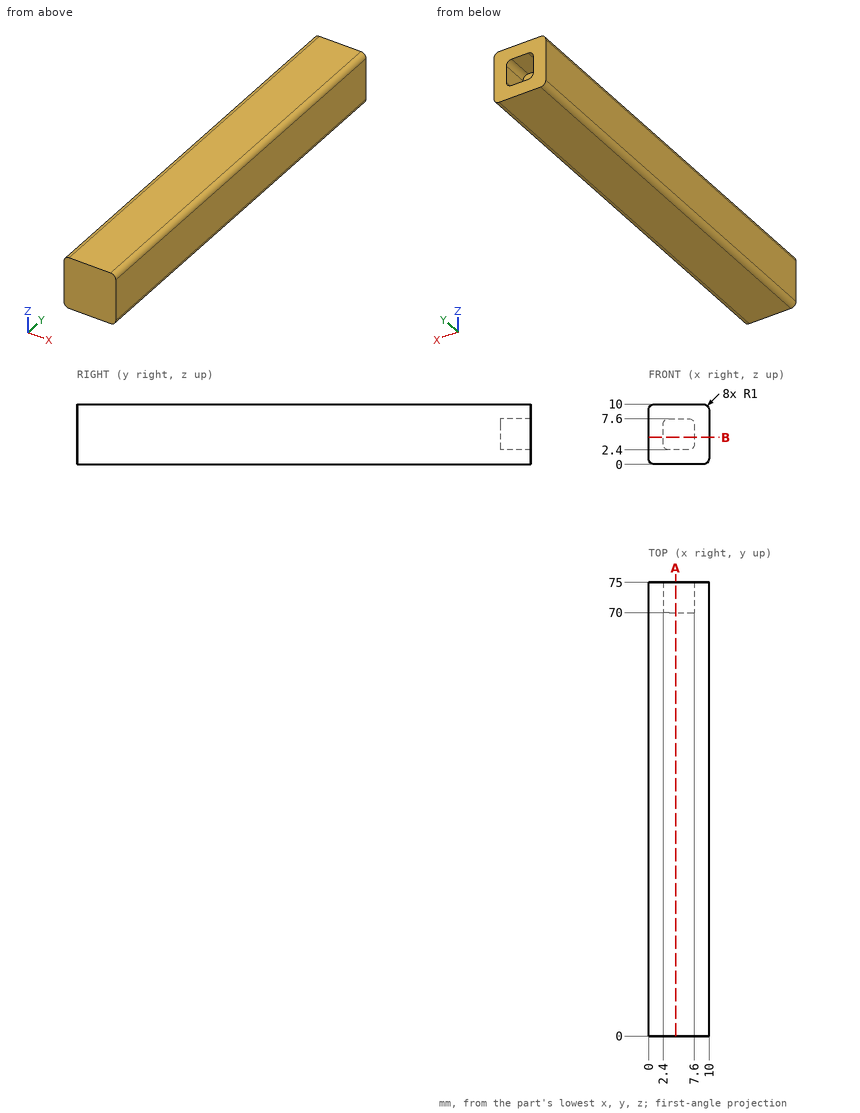
Source: three-view drawing plus pictorial views. Frame: mm from the lowest corner of the part. Round coordinates to 2 decimals unless told otherwise and drop trailing zeros. Loops run counter-clockwise (first coordinate to the right, second up) from the corner with the lowest first, then second, coordinate; pieces in that order, holes last.
Q1. Material intervals for L1, parallel to Y at x = 4.5, z = 5; L2, parallel to X at y = 38, z = 9.5; L3, parallel to Z at x = 9.25, y = 12, sorted ascending.
Q2. Section B-B on z = 4.5. Return loops of the section in (x, y).
Q3. Section A-A on x = 4.5. Return loops of the section in (y, z), plus the area to 3 significant figures.
Evaluation:
1. L1: y = 0 to 70
1. L2: x = 0.13 to 9.87
1. L3: z = 0.03 to 9.97
2. outline: (0, 0) - (10, 0) - (10, 75) - (7.6, 75) - (7.6, 70) - (2.4, 70) - (2.4, 75) - (0, 75) - close
3. outline: (0, 0) - (75, 0) - (75, 2.4) - (70, 2.4) - (70, 7.6) - (75, 7.6) - (75, 10) - (0, 10) - close
3. area: 724 mm2
